Drawing for the job (mm, zero at the part's lowest x, y, z). A direction names the side the tool comes from. Give positions to 0.01 mm unless a question says otherwise; leave off trailing zeros. Write each loop counter-clockwise with the first axis right and the second up, starting at its lowest first coordinate (ties: lowest second). Pieces come first, ordered by that corner, then holes. Notation, with made-up numbers: M 73.25,88 L 82.25,88 A21 ccw 82.25,119 Z; hole C 1.25,84 d11. An arc over 180 degrees is marked long. Use CSV: the item, a comma, the result in double quotes. Start each with the question number.
1. Band-saw the part on A-A, the plane z = 314. List the corners of the cut face in (x, y), then the cut area to 3 significant figures.
2. Band-saw the part on B-B, the plane y = 35.5. List the corners of the cut face in (x, z) (1 decimal).
3. Drop flat-ended pins along their axis: pin 1 Ø18 at (x, y) = (142, 137.5) entering from -Z; pin 2 Ø24 at (x, y) = (170, 148) entering from +Z; pin 3 Ø8 at (y, z) = (136.5, 209.5) entering from -X. Give the stop position or say it passes through.
4. 3-axis set-ups, long thin cutter, end or side, ignore diameter. For the marked faces 5, 6 and 7: which of +Z, -Z, +X, -X, +Y, -Y reach the whole face in a straight line?
5. Band-saw the part on D-D, the plane y = 117.5. List the corners of the cut face in (x, z), then the cut area to 3 significant figures.
6. Band-saw the part on C-C, the plane x = 109. List the corners of the cut face in (y, z) (1 decimal).
7. Drill centre lines: line 1 along Z through (x, y) = (143.5, 162); line 2 along X through (y, z) = (104.5, 257.5); line 3 along Z through (x, y) = (166.5, 102). Where is each one in solid material? Low to high. Write a range as from..to.
8. Mould opens along X. For the marked faces 1, 2, 3 and 4 say: pulls with the +X half, pulls with the -X half, needs draft (parallel to the pull), parting line crosses it, or undercut.
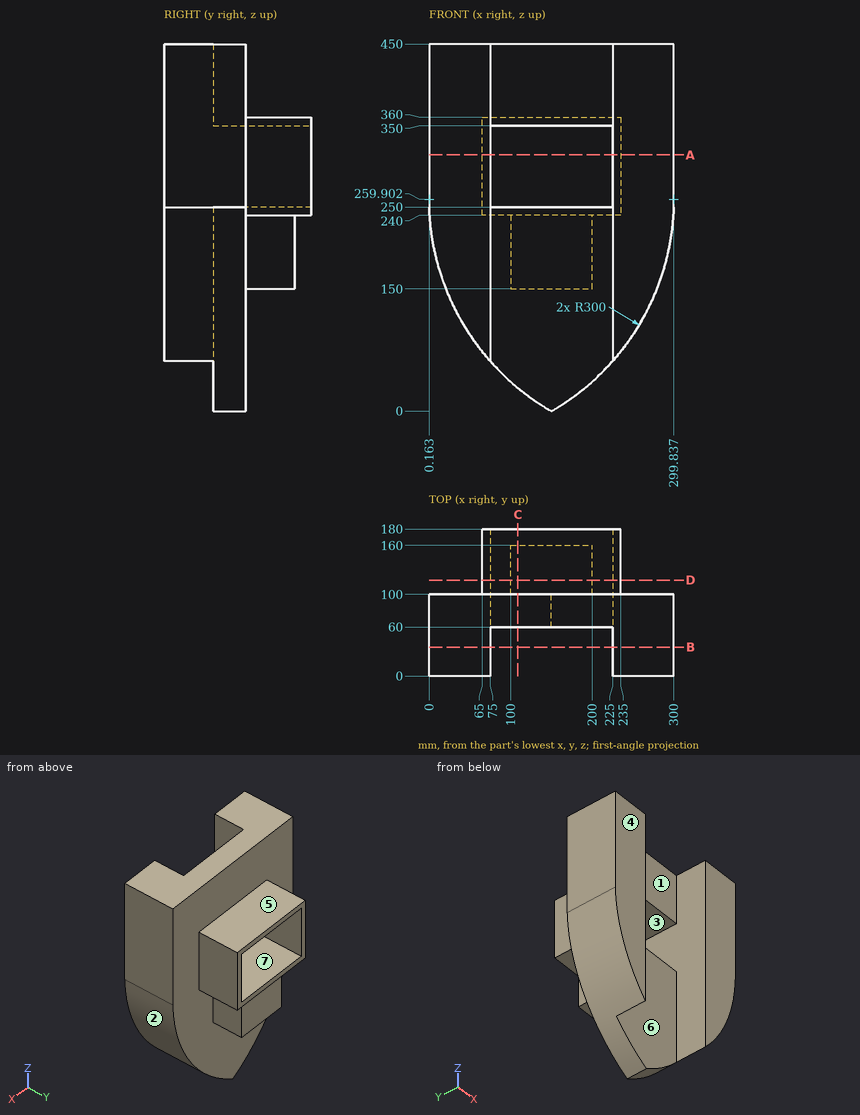
Output:
1,outline,"M 0,0 L 75,0 L 75,180 L 65,180 L 65,100 L 0,100 Z; M 225,0 L 300,0 L 300,100 L 235,100 L 235,180 L 225,180 Z"
1,area,"16,600 mm²"
2,outline,"M 0,250 A300 ccw 75,61.3 L 75,450 L 0,450 Z; M 225,61.3 A300 ccw 300,250 L 300,450 L 225,450 Z"
3,pin 1,"stops at z = 150"
3,pin 2,"stops at z = 360"
3,pin 3,"stops at x = 100"
4,face 5,"+Z, +X, -X, +Y"
4,face 6,"+Z, -Z, -Y"
4,face 7,"+Y, -Y"
5,outline,"M 65,240 L 100,240 L 100,150 L 200,150 L 200,240 L 235,240 L 235,360 L 65,360 Z; hole M 75,250 L 225,250 L 225,350 L 75,350 Z"
5,area,"14,400 mm²"
6,outline,"M 60,28.4 L 100,28.4 L 100,150 L 160,150 L 160,240 L 180,240 L 180,250 L 60,250 Z; M 60,350 L 180,350 L 180,360 L 100,360 L 100,450 L 60,450 Z"
7,line 1,"z = 240..250, 350..360"
7,line 2,"x = 65..75, 225..235"
7,line 3,"z = 150..250, 350..360"
8,face 1,"undercut"
8,face 2,"pulls with the +X half"
8,face 3,"undercut"
8,face 4,"needs draft"
